Here's how the part is built. I have some questions about the finished solid (model axes, mm). A direction names the side the tool comes from. Round coordinates to 2 decimals unless told otherwise and drop trailing zeros. Write each loop counter-clockwise with the first axis right and the second up, starting at its lowest first coordinate (ties: lowest second). Pieces come first, ordered by that corner, then holes. Notation, with made-up numbers: (76, -32) -> (89, -32) arc R33 cw to (89, -4) -> close; hole circle Ø6 at (71, 40). An arc over 180 degrees is marked (long way). Put each result on its own line as item: value. Start each with the question number.
1) If I drill on line 1 along Z through (x, y) = (0, -17.75); line 2 along Z through (x, y) = (0, -22.9); line 3 along Z through (x, y) = (23.5, -20.25), over which ranges is the centre line in solid material (lowest first)? Write a range as [from, to].
2) I want a section at D-D, the plane x = 15. List the corners of the cut face in (y, z) for me (3 decimals).
3) I want a section at A-A, the plane x = 0. List the corners of the cut face in (y, z) for me (3 decimals).
4) I want a section at C-C, the plane y = -3. List the corners of the cut face in (x, z) for me, then the cut area to 3 significant figures.
5) Which directions (+Z, -Z, +X, -X, +Y, -Y) give clear straight access to the entire face, cutting with the end or side of a thin tool? Please do faces 1 (the flat face through (11, -23.774, 14)), 2 (the flat face through (14, -28.575, -14)), 3 (the cylindrical face through (16.72, -14.46, 5.26)).
6) We'd pull the mould along Y, two halves only. Please class faces 4 (the flat face through (8, -6.35, -12)), 5 (the cylindrical face through (17.7, -23.05, -5.57)), 6 (the flat face through (14, 0, -7)): released by +Y, released by -Y, zero draft, split by the parting line, or undercut.
7) Will these pins go through, and if not, where does the flat tip stop? P1, Ø2, axis at x = -19, y = -12.5, coming from the -Z side; P2, Ø11, axis at x = -2.5, z = 7.5, coming from the -Y side; P3, Ø1.5, axis at x = 14, z = 9, coming from the -Y side; P4, Ø3, axis at y = -22.5, z = -24.5, coming from the -X side.
8) I want a section at B-B, the plane z = 0. List the corners of the cut face in (x, y) for me (3 decimals), then the cut area to 3 significant figures.
from build123d import *

# Parameters (mm, degrees)
F0_R           = 31.75
F1_DEPTH       = 28.575
F3_D           = 27.432
F3_CBORE_D     = 35.052
F3_CBORE_DEPTH = 22.225
F4_W           = 11.247322
F4_H           = 1.4224


with BuildPart() as f1:
    # F0 (on Front) → F1 (new body)
    with BuildSketch(Plane.XZ):
        Circle(F0_R)
    extrude(amount=F1_DEPTH)

    # F3 (through all)
    with Locations(Plane.XZ.offset(28.575)):
        with Locations((0, 0)):
            CounterBoreHole(F3_D / 2, F3_CBORE_D / 2, F3_CBORE_DEPTH)

    # F4 (on Top) → F5 (revolve, cut)
    with BuildSketch(Plane.XY):
        with Locations((12.931039, -23.0632)):
            Rectangle(F4_W, F4_H)
    revolve(axis=Axis((0, 2.595396, 0), (0, 1, 0)), mode=Mode.SUBTRACT)


solid = f1.part
Findings:
1. line 1: z = [-31.75, -17.53], [17.53, 31.75]
1. line 2: z = [-31.75, -18.55], [18.55, 31.75]
1. line 3: z = [-21.35, 21.35]
2. outline: (-28.575, -27.983) -> (0, -27.983) -> (0, 27.983) -> (-28.575, 27.983) -> (-28.575, 9.064) -> (-23.774, 9.064) -> (-23.774, 10.921) -> (-22.352, 10.921) -> (-22.352, 9.064) -> (-6.35, 9.064) -> (-6.35, -9.064) -> (-22.352, -9.064) -> (-22.352, -10.921) -> (-23.774, -10.921) -> (-23.774, -9.064) -> (-28.575, -9.064) -> close
3. outline: (-28.575, -31.75) -> (0, -31.75) -> (0, -13.716) -> (-6.35, -13.716) -> (-6.35, -17.526) -> (-22.352, -17.526) -> (-22.352, -18.555) -> (-23.774, -18.555) -> (-23.774, -17.526) -> (-28.575, -17.526) -> close; (-28.575, 17.526) -> (-23.774, 17.526) -> (-23.774, 18.555) -> (-22.352, 18.555) -> (-22.352, 17.526) -> (-6.35, 17.526) -> (-6.35, 13.716) -> (0, 13.716) -> (0, 31.75) -> (-28.575, 31.75) -> close
4. outline: circle Ø63.5 at (0, 0); hole circle Ø27.43 at (0, 0)
4. area: 2,580 mm2
5. face 1: none
5. face 2: +Z, -Z, +X, -X, -Y
5. face 3: -Y
6. face 4: released by -Y
6. face 5: undercut
6. face 6: released by +Y
7. P1: stops at z = -26.15
7. P2: passes through
7. P3: stops at y = -6.35
7. P4: stops at x = -21.89
8. outline: (-31.75, -28.575) -> (-17.526, -28.575) -> (-17.526, -23.774) -> (-18.555, -23.774) -> (-18.555, -22.352) -> (-17.526, -22.352) -> (-17.526, -6.35) -> (-13.716, -6.35) -> (-13.716, 0) -> (-31.75, 0) -> close; (13.716, -6.35) -> (17.526, -6.35) -> (17.526, -22.352) -> (18.555, -22.352) -> (18.555, -23.774) -> (17.526, -23.774) -> (17.526, -28.575) -> (31.75, -28.575) -> (31.75, 0) -> (13.716, 0) -> close
8. area: 858 mm2
